from build123d import *

# Parameters (mm, degrees)
CUT_EXTRUDE1_DEPTH      = 102.550480058
CUT_EXTRUDE1_DEPTH_BACK = 102.550480058
SKETCH3_R               = 5


with BuildPart() as part:
    # Sweep-Thin1: sweep along a path in Sketch1
    with BuildLine(Plane(origin=(0, 0, 0), x_dir=(1, 0, 0), z_dir=(0, 1, 0))) as sweep_thin1_path:
        Line((0, 0), (-100, 0))
    # Sketch2 → Sweep-Thin1 (sweep)
    with BuildSketch(Plane(origin=(0, 0, 0), x_dir=(0, 0, -1), z_dir=(1, 0, 0))):
        with BuildLine():
            Line((4.5, 12.5), (-4.5, 12.5))
            ThreePointArc((-4.5, 12.5), (-10.156854249, 10.156854249), (-12.5, 4.5))
            Line((-12.5, 4.5), (-12.5, -4.5))
            ThreePointArc((-12.5, -4.5), (-10.156854249, -10.156854249), (-4.5, -12.5))
            Line((-4.5, -12.5), (4.5, -12.5))
            ThreePointArc((4.5, -12.5), (10.156854249, -10.156854249), (12.5, -4.5))
            Line((12.5, -4.5), (12.5, 4.5))
            ThreePointArc((12.5, 4.5), (10.156854249, 10.156854249), (4.5, 12.5))
        make_face()
        with BuildLine():
            Line((4.5, 9.5), (-4.5, 9.5))
            ThreePointArc((-4.5, 9.5), (-8.035533906, 8.035533906), (-9.5, 4.5))
            Line((-9.5, 4.5), (-9.5, -4.5))
            ThreePointArc((-9.5, -4.5), (-8.035533906, -8.035533906), (-4.5, -9.5))
            Line((-4.5, -9.5), (4.5, -9.5))
            ThreePointArc((4.5, -9.5), (8.035533906, -8.035533906), (9.5, -4.5))
            Line((9.5, -4.5), (9.5, 4.5))
            ThreePointArc((9.5, 4.5), (8.035533906, 8.035533906), (4.5, 9.5))
        make_face(mode=Mode.SUBTRACT)
    sweep(path=sweep_thin1_path.line)

    # Sketch3 → Cut-Extrude1 (cut, two sides: drawn at the far end of the back side and taken through both)
    with BuildSketch(Plane.XY.offset(-CUT_EXTRUDE1_DEPTH_BACK)):
        with Locations(Location((-50, 0, 0), (0, 0, 64.158067237))):
            Circle(SKETCH3_R)
    extrude(amount=CUT_EXTRUDE1_DEPTH + CUT_EXTRUDE1_DEPTH_BACK, mode=Mode.SUBTRACT)


solid = part.part
Verification items for the finished model (mm, model axes). A direction names the side the tool comes from. Coordinates: 2 decimals unless noted, no trailing zeros. Loops run counter-clockwise (first coordinate to the right, second up) from the corner with the lowest first, then second, coordinate; pieces in that order, holes last. Notation, with made-up numbers: M 55.25,69.25 L 112.25,69.25 A12 cw 112.25,82.25 Z; hole C 59.5,38 d3. An arc over 180 degrees is marked long. One line per item, written item: value.
1. Set-up check for faces 4 (the cylindrical face through (-50.7, -10.094, -10.219)), 5 (the cylindrical face through (-50.7, 8, 8.07)): record each of +Z, -Z, +X, -X, +Y, -Y from which the full face is reachable in a straight line by a thin tool's end or side.
Answers follow:
face 4: -Z, +X, -X, -Y
face 5: +X, -X
2. Material ranges on line 1 along Z through (x, y) = (-44.5, -1.5); line 2 along X through (y, z) = (0, 10.2), recorded low to high. Write a range as from..to.
Answers follow:
line 1: -12.5..-9.5, 9.5..12.5
line 2: -100..-55, -45..0
3. Mould release check, pull along Z, two halves, no side actions. Record for faces 1 (the cylindrical face through (-50.7, 10.219, -10.094)), 2 (the flat face through (-51, -9.5, 0)), 3 (the flat face through (-76, 0, 12.5)): pulls with the +Z half, pulls with the -Z half, needs draft (parallel to the pull), parting line crosses it, or undercut.
Answers follow:
face 1: pulls with the -Z half
face 2: undercut
face 3: pulls with the +Z half
4. Section check D-D on x = -50. Record the cut outline in (y, z).
Answers follow:
outline: M -12.5,-4.5 A8 ccw -5,-12.48 L -5,-9.47 A5 cw -9.5,-4.5 L -9.5,4.5 A5 cw -5,9.47 L -5,12.48 A8 ccw -12.5,4.5 Z; M 5,-12.48 A8 ccw 12.5,-4.5 L 12.5,4.5 A8 ccw 5,12.48 L 5,9.47 A5 cw 9.5,4.5 L 9.5,-4.5 A5 cw 5,-9.47 Z
5. Section check A-A on y = 0. Record the cut outline in (x, z), plus the area to 3 significant figures.
Answers follow:
outline: M -100,-12.5 L -55,-12.5 L -55,-9.5 L -100,-9.5 Z; M -100,9.5 L -55,9.5 L -55,12.5 L -100,12.5 Z; M -45,-12.5 L 0,-12.5 L 0,-9.5 L -45,-9.5 Z; M -45,9.5 L 0,9.5 L 0,12.5 L -45,12.5 Z
area: 540 mm^2
6. Section check C-C on x = -71. Record the cut outline in (y, z), plus the area to 3 significant figures.
Answers follow:
outline: M -12.5,-4.5 A8 ccw -4.5,-12.5 L 4.5,-12.5 A8 ccw 12.5,-4.5 L 12.5,4.5 A8 ccw 4.5,12.5 L -4.5,12.5 A8 ccw -12.5,4.5 Z; hole M -9.5,-4.5 A5 ccw -4.5,-9.5 L 4.5,-9.5 A5 ccw 9.5,-4.5 L 9.5,4.5 A5 ccw 4.5,9.5 L -4.5,9.5 A5 ccw -9.5,4.5 Z
area: 231 mm^2
7. Gauge pin test, flat ends, axial feed: P1, Ø2, axis at x = -14.5, y = -6.5, coming from the +Z side; P2, Ø9, axis at x = -50, y = 0, coming from the -Z side; P3, Ø10, axis at x = -67, z = -9, coming from the -Y side; P4, Ø2, axis at x = -74.5, y = -9.5, coming from the -Z side. Record the tip position at first contact, or that the pin passes through.
Answers follow:
P1: z = 12.44
P2: through
P3: y = -12.5
P4: z = -11.43
8. Section check B-B on z = -2. Record the cut outline in (x, y).
Answers follow:
outline: M -100,-12.5 L 0,-12.5 L 0,-9.5 L -100,-9.5 Z; M -100,9.5 L 0,9.5 L 0,12.5 L -100,12.5 Z
